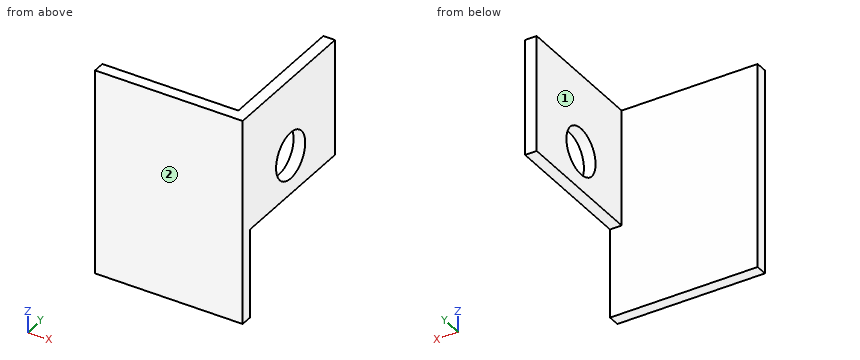
Autodesk Inventor part; units mm, degrees
ref_plane "YZ Plane" through (0, 0, 0) normal (1, 0, 0) x (0, 1, 0)
ref_plane "XZ Plane" through (0, 0, 0) normal (0, 1, 0) x (-1, 0, 0)
ref_plane "XY Plane" through (0, 0, 0) normal (0, 0, 1) x (1, 0, 0)
sketch "Sketch1" plane through (0, 0, 0) normal (0, 0, 1) x (1, 0, 0)
  point P0 (0, 0)
sketch "Sketch2" plane through (0, 0, 0) normal (0, 0, 1) x (1, 0, 0)
  line L0 (0, 0) -> (76, 0)
  line L1 (76, 0) -> (76, 76)
  line L2 (76, 76) -> (0, 76)
  line L3 (0, 76) -> (0, 0)
  line L4 (70, 6) -> (6, 6)
  line L5 (6, 6) -> (6, 70)
  line L6 (6, 70) -> (70, 70)
  line L7 (70, 70) -> (70, 6)
  line L8 (6, 6) -> (0, 6)
  line L9 (70, 70) -> (70, 76)
  dimension "d0" = 76
  dimension "d1" = 76
  dimension "d2" = 6
extrude "Extrusion1" add sketch "Sketch2" against normal blind 106 contours L3 L8 L4 L7 L9 L2 L1 L0
sketch "Sketch3" plane through (76, 76, 0) normal (1, 0, 0) x (0, 0, -1)
  line L0 (106, 0) -> (106, -76)
  line L1 (0, 0) -> (106, 0)
  line L2 (0, -76) -> (0, 0)
  circle A0 centre (40, -36.5) radius 12
  line L3 (0, -76) -> (106, -76)
  dimension "d6" = 24
  dimension "d7" = 40
extrude "Extrusion2" cut sketch "Sketch3" against normal blind 76 contours A0
sketch "Sketch5" plane through (70, 76, -106) normal (-1, 0, 0) x (0, 0, 1)
  line L0 (0, -70) -> (106, -70)
  line L1 (106, 0) -> (0, 0)
  line L2 (106, -70) -> (46, -70)
  line L3 (46, -70) -> (46, 0)
  line L4 (46, 0) -> (106, 0)
  line L5 (106, 0) -> (106, -70)
  line L6 (0, -70) -> (0, 0)
  line L7 (0, 0) -> (46, 0)
  line L8 (46, 0) -> (46, -70)
  line L9 (46, -70) -> (0, -70)
  line L10 (0, -70) -> (0, 0)
  point P0 (106, -76)
  dimension "d23" = 60
extrude "Extrusion3" cut sketch "Sketch5" against normal blind 10 contours L6 L1 L3 L0
properties part number "P005" material "Aluminum 6061"
Can you work these out from the model? Positions are in its coordinate system, mm. Face numbers are marked on the shaded views. A direction names the side the tool comes from. Round coordinates to 2 decimals unless told otherwise and drop trailing zeros. Order: outer loops, then holes, each group sorted by start corner. A loop starts at its lowest first (then second) coordinate and runs counter-clockwise, first axis right, second up. Notation, with made-up numbers: (10.5, 30.5) -> (64.5, 30.5) arc R7 cw to (64.5, 43.5) -> close; hole circle Ø1 at (21.5, 59). An arc over 180 degrees is marked (long way). Return JSON: item names as keys, results as strings. Group by question number.
1. If we section it at C-C, the plane z = -40: Write out the boundary of the cut face in (x, y), then the cut area to 3 significant figures.
2. If we section it at D-D, the plane z = -77.5: Write out the boundary of the cut face in (x, y), then the cut area to 3 significant figures.
3. If we section it at B-B, the plane x = 71.5: Write out the boundary of the cut face in (y, z).
4. Which directions (+Z, -Z, +X, -X, +Y, -Y) give clear straight access to the entire face, cutting with the end or side of a thin tool? Please do the marked faces 1 and 2.
5. If we section it at A-A, the plane y = 39.5: Write out the boundary of the cut face in (x, z).
6. Will these pins go through, and if not, where does the flat tip stop? pin 1 (5 mm diameter, centred on x = 74.5, y = 34, fed in from -Z); pin 2 (1.5 mm diameter, centred on y = 62.5, z = -56.5, fed in from -X).
7. I need wall thicknesses on line 1 (Y direction, x = 74.4, z = -40); line 2 (X direction, y = 49.5, z = -10); line 3 (Y direction, x = 16, z = -35.5). Which ranges of each line are inside material? Lowest first, please. Write a range as [from, to].
Output values:
{
 "1": {"outline": "(0, 0) -> (76, 0) -> (76, 27.5) -> (70, 27.5) -> (70, 6) -> (0, 6) -> close; (70, 51.5) -> (76, 51.5) -> (76, 76) -> (70, 76) -> close", "area": "732 mm²"},
 "2": {"outline": "(0, 0) -> (76, 0) -> (76, 6) -> (0, 6) -> close", "area": "456 mm²"},
 "3": {"outline": "(0, -106) -> (6, -106) -> (6, -60) -> (76, -60) -> (76, 0) -> (0, 0) -> close; hole circle Ø24 at (39.5, -40)"},
 "4": {"face 1": "+Z, -Z, -X, +Y", "face 2": "+Z, -Z, +X, -X, -Y"},
 "5": {"outline": "(70, -60) -> (76, -60) -> (76, -52) -> (70, -52) -> close; (70, -28) -> (76, -28) -> (76, 0) -> (70, 0) -> close"},
 "6": {"pin 1": "z = -60", "pin 2": "x = 70"},
 "7": {"line 1": "[0, 27.5], [51.5, 76]", "line 2": "[70, 76]", "line 3": "[0, 6]"}
}
